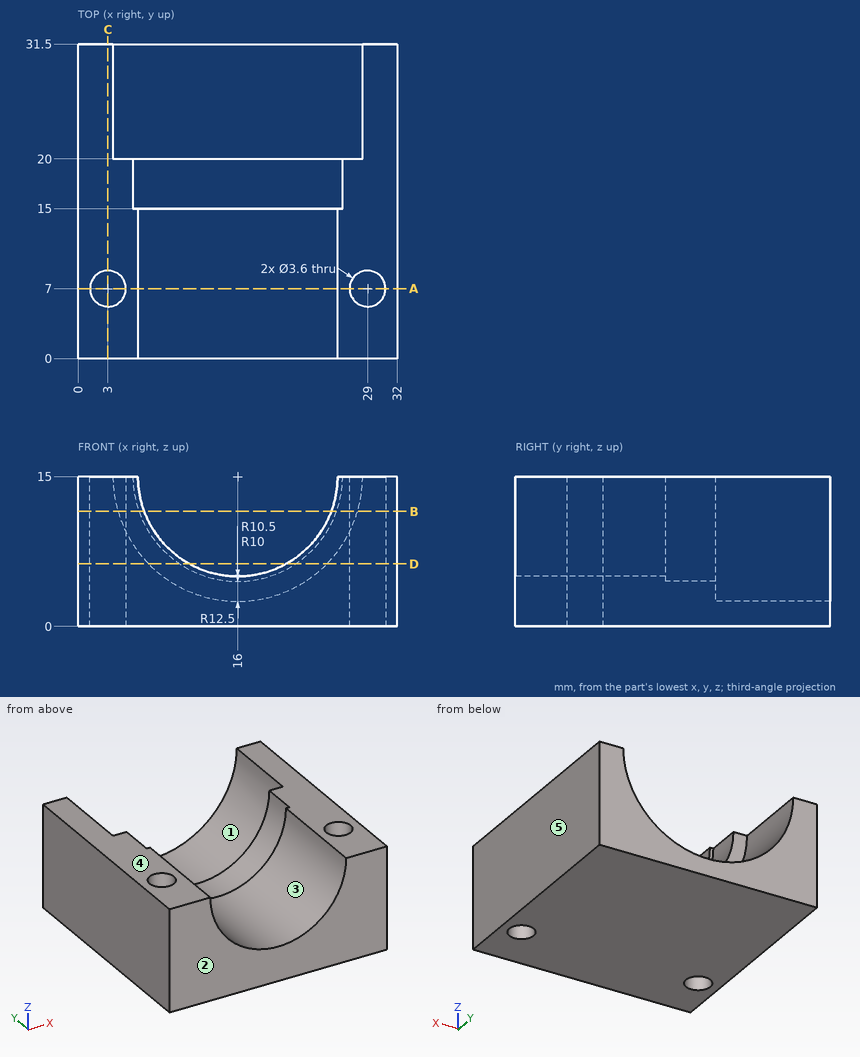
Geometry check sheet. Reference: drawing and pictorial views, mm from the part's lowest x, y, z. A direction names the side the tool comes from. Give positions to 0.01 mm unless a question says otherwise; leave off trailing zeros. Order: outer loops, then holes, each group sorted by start corner. A loop starts at its lowest first (then second) coordinate and runs counter-clockwise, first axis right, second up. Notation, with made-up numbers: M 39.5,-18.75 L 96.5,-18.75 A21 cw 96.5,3.25 Z; hole C -35.5,19 d2. An arc over 180 degrees is marked long. Use one line per item in the form item = value. Start each with the question number.
Q1. Section check D-D (z = 6.25). Enter the section's corners in (x, y), then the cut area to 3 significant figures.
Q2. Section check A-A (y = 7). Enter the section's corners in (x, z), then the cut area to 3 significant figures.
Q3. Scan lines: line 1 along Y through (x, z) = (29, 5); line 2 along X through (y, z) = (6, 4.25); line 3 along Z through (x, y) = (16, 11.5). Record each from-to range of solid material in increasing order. Write a range as [from, to].
Q4. Access from +Z, -Z, +X, -X, +Y, -Y to the whole of each face (thin tool, end or side, straight path). Record for the marked faces 1 and 2.
Q5. Section check C-C (x = 3). Enter the section's corners in (y, z), then the cut area to 4 significant figures.
Q6. Section check B-B (z = 11.5). Enter the section's corners in (x, y), then the cut area to 3 significant figures.
Q7. Mould release check, pull along X, two halves, no side actions. Record for the marked faces 3, 4 and 5: +X half, -X half, draft (parallel to the pull), parting line (faces both ways), or undercut.
Q8. Go/stop test with flat-tipped pins: pin 1 Ø12 at (x, y) = (18.5, 15.5) entering from -Z; pin 2 Ø1.5 at (x, y) = (10.5, 12.5) entering from +Z. Record where each tip stops, or that it passes through.
Evaluation:
q1.outline = M 0,0 L 11.16,0 L 11.16,15 L 10.2,15 L 10.2,20 L 7.07,20 L 7.07,31.5 L 0,31.5 Z; M 20.84,0 L 32,0 L 32,31.5 L 24.93,31.5 L 24.93,20 L 21.8,20 L 21.8,15 L 20.84,15 Z; hole C 3,7 d3.6; hole C 29,7 d3.6
q1.area = 579 mm2
q2.outline = M 0,0 L 1.2,0 L 1.2,15 L 0,15 Z; M 4.8,0 L 27.2,0 L 27.2,15 L 26,15 A10 cw 6,15 L 4.8,15 Z; M 30.8,0 L 32,0 L 32,15 L 30.8,15 Z
q2.area = 215 mm2
q3.line_1 = [0, 5.2], [8.8, 31.5]
q3.line_2 = [0, 1.5], [4.5, 27.5], [30.5, 32]
q3.line_3 = [0, 5]
q4.face_1 = +Z, +Y
q4.face_2 = +Z, -Z, +X, -X, -Y
q5.outline = M 0,0 L 5.2,0 L 5.2,15 L 0,15 Z; M 8.8,0 L 31.5,0 L 31.5,15 L 8.8,15 Z
q5.area = 418.5 mm2
q6.outline = M 0,0 L 6.63,0 L 6.63,15 L 6.1,15 L 6.1,20 L 4,20 L 4,31.5 L 0,31.5 Z; M 25.37,0 L 32,0 L 32,31.5 L 28,31.5 L 28,20 L 25.9,20 L 25.9,15 L 25.37,15 Z; hole C 3,7 d3.6; hole C 29,7 d3.6
q6.area = 332 mm2
q7.face_3 = undercut
q7.face_4 = draft
q7.face_5 = +X half
q8.pin_1 = 0
q8.pin_2 = 7.19
